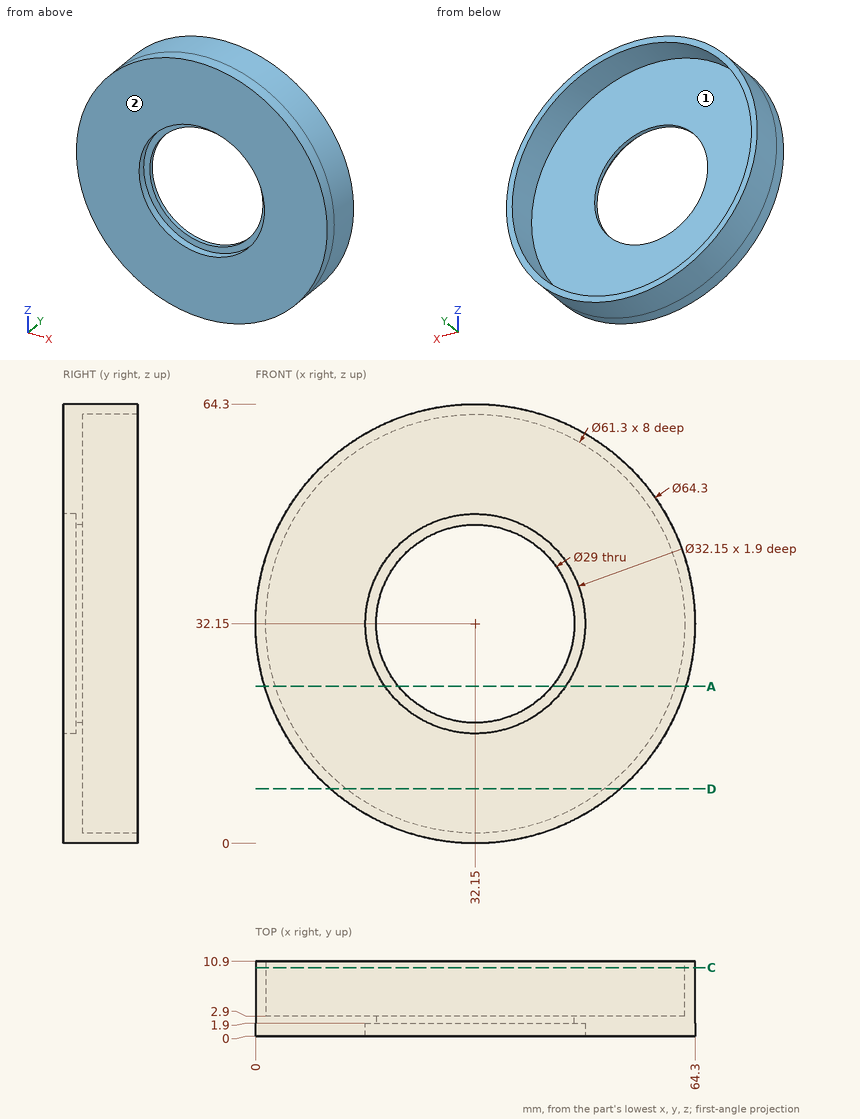
For this review, use the dimensioned drawing (mm, ordinates from the lowest corner) and the shaded views. Coordinates: 2 decimals unless noted, no trailing zeros. Order: outer loops, then holes, each group sorted by start corner. A loop starts at its lowest first (then second) coordinate and runs counter-clockwise, first axis right, second up. Notation, with made-up numbers: (81, 14.5) - (114, 14.5) arc R22 ccw to (114, 29.5) - close; hole circle Ø10 at (36, 60.5). An arc over 180 degrees is marked (long way). Answer as a JSON object with one key per item and string values. Group by question number.
1. We need section A-A on z = 23. State the section outline as (x, y) points.
2. Clearance check with flat-ended pins moving along their axes: P1, Ø23, axis at x = 32.15, z = 32.15, coming from the +Y side; P2, Ø1, axis at x = 12, y = 1.5, coming from the -Z side; P3, Ø1.5, axis at y = 3, z = 40.5, coming from the +X side; P4, Ø5, axis at x = 26.5, y = 3.5, coming from the +Z side. State where each tip first meets the part, or that it passes through.
3. We need section C-C on y = 10. State the section outline as (x, z) points, then the cut area to 3 significant figures.
4. For probe 1 along Z at (x, y) = (32.15, 0.8) (3 decimals); probe 2 along Z at (x, y) = (32.15, 2.7), list the stretches that pass through material, from the lowest coordinate up.
5. We need section D-D on z = 8. State the section outline as (x, y) points, then the cut area to 3 significant figures.
6. The part is to be moulded in two halves that separate along Z. For the marked faces 1 and 2, say which applies: pulls with the +Z half, pulls with the -Z half, needs draft (parallel to the pull), parting line crosses it, or undercut.
Final values:
{
 "1": {"outline": "(1.33, 0) - (18.93, 0) - (18.93, 1.9) - (20.9, 1.9) - (20.9, 2.9) - (2.9, 2.9) - (2.9, 10.9) - (1.33, 10.9) - close; (43.4, 1.9) - (45.37, 1.9) - (45.37, 0) - (62.97, 0) - (62.97, 10.9) - (61.4, 10.9) - (61.4, 2.9) - (43.4, 2.9) - close"},
 "2": {"P1": "through", "P2": "z = 6.7", "P3": "x = 63.39", "P4": "z = 64.15"},
 "3": {"outline": "circle Ø64.3 at (32.15, 32.15); hole circle Ø61.3 at (32.15, 32.15)", "area": "296 mm²"},
 "4": {"probe 1": "0 to 16.075, 48.225 to 64.3", "probe 2": "0 to 17.65, 46.65 to 64.3"},
 "5": {"outline": "(10.93, 0) - (53.37, 0) - (53.37, 10.9) - (51.02, 10.9) - (51.02, 2.9) - (13.28, 2.9) - (13.28, 10.9) - (10.93, 10.9) - close", "area": "161 mm²"},
 "6": {"face 1": "undercut", "face 2": "needs draft"}
}
